Part model, mm, in its own coordinate system. Face numbers are marked on the shaded views. A direction names the side the tool comes from. Coordinates: 2 decimals unless noted, no trailing zeros. Write each loop counter-clockwise with the first axis right and the second up, starting at its lowest first coordinate (ties: lowest second). Pieces come first, ordered by that corner, then holes. Notation, with made-up numbers: (63, 20.25) - (86, 20.25) arc R6 ccw to (86, 24.25) - close; hole circle Ø3 at (15.5, 71). An arc over 180 degrees is marked (long way). Use a Markdown table: item, result.
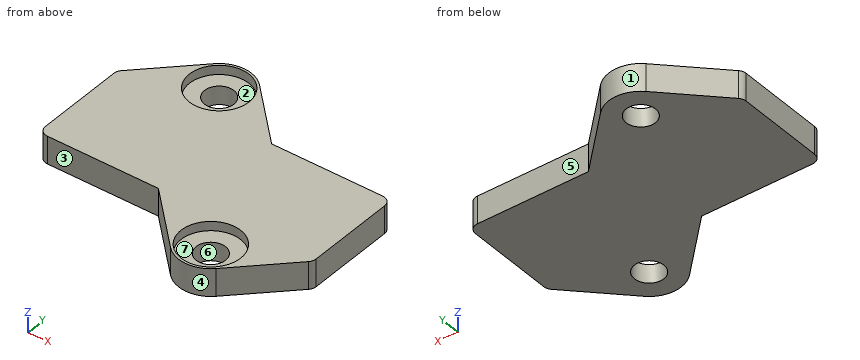
```python
from build123d import *

# Parameters (mm, degrees)
EXTRUDE_1_DEPTH     = 3
SKETCH_3_R          = 3.25
CUT_EXTRUDE_1_DEPTH = 1
FILLET_1_R          = 1
SKETCH_6_R          = 1.6
CUT_EXTRUDE_3_DEPTH = 20.754746265


with BuildPart() as part:
    # 草图1 → 凸台-拉伸1 (new body)
    with BuildSketch(Plane.XY):
        with BuildLine():
            Line((15, 5.5), (1.899494937, 5.5))
            Line((1.899494937, 5.5), (-4.075378798, 11.474873734))
            ThreePointArc((-4.075378798, 11.474873734), (-6.550252532, 12.5), (-9.025126266, 11.474873734))
            Line((-9.025126266, 11.474873734), (-15, 5.5))
            Line((-15, 5.5), (-15, -5.5))
            Line((-15, -5.5), (-1.899494937, -5.5))
            Line((-1.899494937, -5.5), (4.075378798, -11.474873734))
            ThreePointArc((4.075378798, -11.474873734), (6.550252532, -12.5), (9.025126266, -11.474873734))
            Line((9.025126266, -11.474873734), (15, -5.5))
            Line((15, -5.5), (15, 5.5))
        make_face()
    extrude(amount=EXTRUDE_1_DEPTH)

    # 草图3 → 切除-拉伸1 (cut)
    with BuildSketch(Plane.XY.offset(3)):
        with Locations((-6.550252532, 9)):
            Circle(SKETCH_3_R)
        with Locations((6.550252532, -9)):
            Circle(SKETCH_3_R)
    extrude(amount=-CUT_EXTRUDE_1_DEPTH, mode=Mode.SUBTRACT)

    # 圆角1
    fillet_1_edges = [part.edges().sort_by_distance(p)[0] for p in [
        (15, -5.5, 1.5),
        (-15, -5.5, 1.5),
        (-15, 5.5, 1.5),
        (15, 5.5, 1.5),
    ]]
    fillet(fillet_1_edges, radius=FILLET_1_R)

    # 草图6 → 切除-拉伸3 (cut, through all)
    with BuildSketch(Plane.XY.offset(3)):
        with Locations((-6.550252532, 9)):
            Circle(SKETCH_6_R)
        with Locations((6.550252532, -9)):
            Circle(SKETCH_6_R)
    extrude(amount=-CUT_EXTRUDE_3_DEPTH, mode=Mode.SUBTRACT)


solid = part.part
```
Item 1: Band-saw the part on B-B, the plane y = 8. Give the cut face in (x, z), then the cut area to 3 significant figures.
From the geometry:
| item | result |
|---|---|
| outline | (-12.5, 0) - (-7.8, 0) - (-7.8, 2) - (-9.64, 2) - (-9.64, 3) - (-12.5, 3) - close; (-5.3, 0) - (-0.6, 0) - (-0.6, 3) - (-3.46, 3) - (-3.46, 2) - (-5.3, 2) - close |
| area | 24.5 mm^2 |
Item 2: Band-saw the part on D-D, the plane x = 3.75. Give the cut face in (y, z), then the cut area to 3 significant figures.
From the geometry:
| item | result |
|---|---|
| outline | (-11.15, 0) - (5.5, 0) - (5.5, 3) - (-7.35, 3) - (-7.35, 2) - (-10.65, 2) - (-10.65, 3) - (-11.15, 3) - close |
| area | 46.6 mm^2 |
Item 3: Two-plate mould, pull along X, no slides. Class the marked faces 4, 5, 6 and 7: pulls with the +X half, pulls with the -X half, needs draft (parallel to the pull), parting line crosses it, or undercut.
From the geometry:
| item | result |
|---|---|
| face 4 | parting line crosses it |
| face 5 | needs draft |
| face 6 | undercut |
| face 7 | undercut |
Item 4: Drop flat-ended pins along their axis: P1, Ø5, axis at x = -3, y = -9.5, coming from the +Z side; P2, Ø1, axis at x = -5.5, z = 2, coming from the +Y side; P3, Ø1.5, axis at x = -6.5, z = 1, coming from the -Y side; P4, Ø6, axis at x = 6.55, y = -9, coming from the +Z side. Give the stop position or say it passes through.
From the geometry:
| item | result |
|---|---|
| P1 | through |
| P2 | y = 12.46 |
| P3 | y = -5.5 |
| P4 | z = 2 |
Item 5: Drill centre lines: probe 1 along Y at (x, z) = (-7.75, 2.2); probe 2 along X at (y, z) = (-10.25, 0.85); probe 3 along Y at (x, z) = (6.5, 2.95). Where is each one in solid material? Low to high.
From the geometry:
| item | result |
|---|---|
| probe 1 | -5.5 to 5.98, 12.02 to 12.29 |
| probe 2 | 2.85 to 5.55, 7.55 to 10.25 |
| probe 3 | -12.5 to -12.25, -5.75 to 5.5 |
Item 6: Band-saw the part on A-A, the plane z = 1.5. Give the cut face in (x, y).
From the geometry:
| item | result |
|---|---|
| outline | (-15, -4.5) arc R1 ccw to (-14, -5.5) - (-1.9, -5.5) - (4.08, -11.47) arc R3.5 ccw to (9.03, -11.47) - (14.71, -5.79) arc R1 ccw to (15, -5.09) - (15, 4.5) arc R1 ccw to (14, 5.5) - (1.9, 5.5) - (-4.08, 11.47) arc R3.5 ccw to (-9.03, 11.47) - (-14.71, 5.79) arc R1 ccw to (-15, 5.09) - close; hole circle Ø3.2 at (-6.55, 9); hole circle Ø3.2 at (6.55, -9) |
Item 7: Band-saw the part on C-C, the plane x = 7. Give the cut face in (y, z), then the cut area to 3 significant figures.
From the geometry:
| item | result |
|---|---|
| outline | (-12.47, 0) - (-10.54, 0) - (-10.54, 2) - (-12.22, 2) - (-12.22, 3) - (-12.47, 3) - close; (-7.46, 0) - (5.5, 0) - (5.5, 3) - (-5.78, 3) - (-5.78, 2) - (-7.46, 2) - close |
| area | 41.3 mm^2 |
Item 8: Which spindle directions (+Z, -Z, +X, -X, +Y, -Y) get a long thin tool onto all of the face, cutting with end or side? Do the marked faces 1, 2 and 3. Say none if no direction does.
From the geometry:
| item | result |
|---|---|
| face 1 | +Z, -Z, +Y |
| face 2 | +Z |
| face 3 | +Z, -Z, -X, -Y |
